Verification items for the finished model (mm, model axes). A direction names the side the tool comes from. Give positions to 0.01 mm unless a question says otherwise; leave off trailing zeros. Write each loop counter-clockwise with the first axis right and the second up, starting at its lowest first coordinate (ties: lowest second). Pieces come first, ordered by that corner, then holes. Notation, with made-up numbers: (36.5, 63) -> (85.5, 63) arc R11 cw to (85.5, 78) -> close; hole circle Ø4 at (-26, -14). An arc over 180 degrees is marked (long way). Write item = value, one per line.
from build123d import *

# Parameters (mm, degrees)
SKETCH1_W          = 172
SKETCH1_H          = 3
SKETCH3_R          = 1.75
SKETCH3_R_2        = 1.6
CUT_EXTRUDE1_DEPTH = 2


with BuildPart() as part:
    # Sketch1 → Revolve1 (revolve)
    with BuildSketch(Plane.XY, mode=Mode.PRIVATE) as revolve1_sk:
        with Locations((-72.807280427, 0.402439024)):
            Rectangle(SKETCH1_W, SKETCH1_H)
    revolve(revolve1_sk.sketch.rotate(Axis((-158.807280427, 1.902439024, 0), (1, 0, 0)), 270), axis=Axis((-158.807280427, 1.902439024, 0), (1, 0, 0)))

    # Sketch3 → Cut-Extrude1 (cut)
    with BuildSketch(Plane(origin=(-158.807280427, 4.902439024, 0), x_dir=(1, 0, 0), z_dir=(0, 1, 0))):
        with Locations(Location((83.8, 0, 0), (0, 0, 270))):
            Circle(SKETCH3_R)
        with Locations(Location((41.5, 0, 0), (0, 0, 270))):
            Circle(SKETCH3_R_2)
        with Locations(Location((53.3, 0, 0), (0, 0, 270))):
            Circle(SKETCH3_R)
        with Locations(Location((130.5, 0, 0), (0, 0, 270))):
            Circle(SKETCH3_R_2)
    extrude(amount=-CUT_EXTRUDE1_DEPTH, mode=Mode.SUBTRACT)


solid = part.part
Item 1: Go/stop test with flat-tipped pins: P1, Ø3.5, axis at x = -28.5, z = 0, coming from the +Y side; P2, Ø1.9, axis at x = -117.31, z = 0, coming from the +Y side; P3, Ø2, axis at x = -80, z = 2, coming from the -Y side; P4, Ø2, axis at x = -123.5, y = 0, coming from the -Z side. Record where each tip stops, or that it passes through.
Response values:
P1 = 4.9
P2 = 2.9
P3 = -0.93
P4 = -2.86
Item 2: Mould release check, pull along X, two halves, no side actions. Record for faces 3 (the cylindrical face through (-104.03, 3.69, 0.94)), 4 (the flat face through (13.193, 2, 0)), 5 (the cylindrical face through (-71.6, 1, 2.86)): +X half, -X half, draft (parallel to the pull), parting line (faces both ways), or undercut.
Response values:
face_3 = undercut
face_4 = +X half
face_5 = draft
Item 3: Sectioned sample at C-C on y = 0.25. Record the cut outline in (x, z).
Response values:
outline = (-158.81, -2.5) -> (13.19, -2.5) -> (13.19, 2.5) -> (-158.81, 2.5) -> close
Item 4: Set-up check for faces 1 (the flat face through (-75, 2.902, 0)), 2 (the flat face through (-158.807, 2, 0)): record each of +Z, -Z, +X, -X, +Y, -Y from which the full face is reachable in a straight line by a thin tool's end or side.
Response values:
face_1 = +Y
face_2 = +Z, -Z, -X, +Y, -Y
Item 5: Material ranges on line 1 (X direction, y = 4.05, z = 0); line 2 (Y direction, x = -78.5, z = -0.25); line 3 (Z direction, x = -43.5, y = 1), recorded low to high.
Response values:
line_1 = -158.81 to -118.91, -115.71 to -107.26, -103.76 to -76.76, -73.26 to -29.91, -26.71 to 13.19
line_2 = -1.09 to 4.89
line_3 = -2.86 to 2.86
Item 6: Sectioned sample at A-A on z = 0. Record the cut outline in (x, y), then the cut area to 3 significant figures.
Response values:
outline = (-158.81, -1.1) -> (13.19, -1.1) -> (13.19, 4.9) -> (-26.71, 4.9) -> (-26.71, 2.9) -> (-29.91, 2.9) -> (-29.91, 4.9) -> (-73.26, 4.9) -> (-73.26, 2.9) -> (-76.76, 2.9) -> (-76.76, 4.9) -> (-103.76, 4.9) -> (-103.76, 2.9) -> (-107.26, 2.9) -> (-107.26, 4.9) -> (-115.71, 4.9) -> (-115.71, 2.9) -> (-118.91, 2.9) -> (-118.91, 4.9) -> (-158.81, 4.9) -> close
area = 1,010 mm^2
Item 7: Sectioned sample at B-B on x = -69. Record the cut outline in (y, z).
Response values:
outline = circle Ø6 at (1.9, 0)
